The figure shows three views and two pictorial views of one solid part (mm, origin at its lowest corner). Answer the questions. A direction names the side the tool comes from. Round coordinates to 2 decimals unless told otherwise and drop trailing zeros. Write each loop counter-clockwise with the first axis right and the second up, starting at its lowest first coordinate (ties: lowest second). Pieces come first, ordered by that corner, then holes. Notation, with made-up numbers: M -25.75,5.5 L 24.25,5.5 A15 cw 24.25,24.5 Z; hole C -6.5,-9.5 d10. An arc over 180 degrees is marked long. Answer in a Markdown table with one row per item.
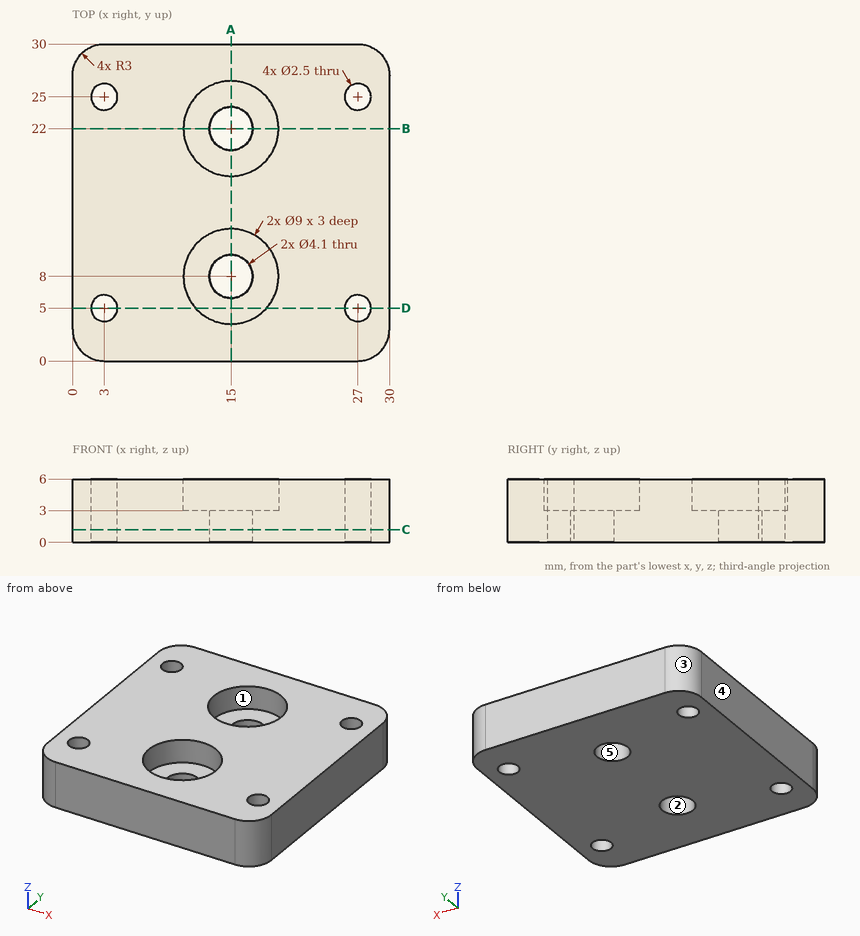
1. The part is cut by section A-A (x = 15). Determine the outline of the cut face in (y, z).
Calculated:
| item | result |
|---|---|
| outline | M 0,0 L 5.95,0 L 5.95,3 L 3.5,3 L 3.5,6 L 0,6 Z; M 10.05,0 L 19.95,0 L 19.95,3 L 17.5,3 L 17.5,6 L 12.5,6 L 12.5,3 L 10.05,3 Z; M 24.05,0 L 30,0 L 30,6 L 26.5,6 L 26.5,3 L 24.05,3 Z |
2. Consider line 1 along Y through (x, z) = (15, 4.7); line 2 along Y through (x, z) = (3, 2.85); line 3 along X through (y, z) = (8, 1.5). Determine where each line is inside the solid, lowest interval first. Write a range as from..to.
Calculated:
| item | result |
|---|---|
| line 1 | y = 0..3.5, 12.5..17.5, 26.5..30 |
| line 2 | y = 0..3.75, 6.25..23.75, 26.25..30 |
| line 3 | x = 0..12.95, 17.05..30 |
3. Given pin 1 (3.5 mm diameter, centred on x = 15, y = 8, fed in from -Z), flat-ended and moving along its own axis, determine where the tip first touches the part or whether it passes through.
Calculated:
| item | result |
|---|---|
| pin 1 | passes through |
4. The part is cut by section D-D (y = 5). Determine the outline of the cut face in (x, z), plus the area to 3 significant figures.
Calculated:
| item | result |
|---|---|
| outline | M 0,0 L 1.75,0 L 1.75,6 L 0,6 Z; M 4.25,0 L 25.75,0 L 25.75,6 L 18.35,6 L 18.35,3 L 11.65,3 L 11.65,6 L 4.25,6 Z; M 28.25,0 L 30,0 L 30,6 L 28.25,6 Z |
| area | 130 mm² |
5. The part is cut by section C-C (z = 1.2). Determine the outline of the cut face in (x, y), plus the area to 3 significant figures.
Calculated:
| item | result |
|---|---|
| outline | M 0,3 A3 ccw 3,0 L 27,0 A3 ccw 30,3 L 30,27 A3 ccw 27,30 L 3,30 A3 ccw 0,27 Z; hole C 3,5 d2.5; hole C 3,25 d2.5; hole C 15,8 d4.1; hole C 15,22 d4.1; hole C 27,5 d2.5; hole C 27,25 d2.5 |
| area | 846 mm² |
6. Determine the mould class of the marked faces 3, 4 and 5 for opening direction Y: released by +Y, released by -Y, zero draft, split by the parting line, or undercut.
Calculated:
| item | result |
|---|---|
| face 3 | released by +Y |
| face 4 | zero draft |
| face 5 | undercut |
7. A tool of negligible diameter and unlimited length cuts with its end or side. For the marked faces 1 and 2, from which of +Z, -Z, +X, -X, +Y, -Y can it reach the whole face along a straight path? Write none if from no direction.
Calculated:
| item | result |
|---|---|
| face 1 | +Z |
| face 2 | +Z, -Z |
8. The part is cut by section B-B (y = 22). Determine the outline of the cut face in (x, z), plus the area to 3 significant figures.
Calculated:
| item | result |
|---|---|
| outline | M 0,0 L 12.95,0 L 12.95,3 L 10.5,3 L 10.5,6 L 0,6 Z; M 17.05,0 L 30,0 L 30,6 L 19.5,6 L 19.5,3 L 17.05,3 Z |
| area | 141 mm² |
